Geometry check sheet. Reference: the model listing, model coordinates, mm. A direction names the side the tool comes from. Coordinates: 2 decimals unless noted, no trailing zeros. Write each loop counter-clockwise with the first axis right and the second up, starting at its lowest first coordinate (ties: lowest second). Pieces come first, ordered by that corner, then holes. Notation, with made-up numbers: (64.5, -14.75) -> (84.5, -14.75) arc R23 cw to (84.5, 24.25) -> close; hole circle Ø8 at (-20.75, 84). An arc over 180 degrees is marked (long way). Put each result on its own line as item: value. Start each with the question number.
from build123d import *

# Parameters (mm, degrees)
SKETCH1_W               = 21.5
SKETCH1_H               = 5
BOSS_EXTRUDE1_DEPTH     = 10
CUT_EXTRUDE1_DEPTH      = 75.426137882
CUT_EXTRUDE1_DEPTH_BACK = 75.426137882
SKETCH2_R               = 1.836585915
SKETCH3_W               = 21.5
SKETCH3_H               = 5
CUT_EXTRUDE2_DEPTH      = 10


with BuildPart() as part:
    # Sketch1 → Boss-Extrude1 (new body)
    with BuildSketch(Plane(origin=(0, 0, 0), x_dir=(0, 0, -1), z_dir=(1, 0, 0))):
        Polygon((-39, 10.5), (-39, -10.5), (39, -10.5), (39, 10.5), (34, 10.5), (34, -0.5), (34, -5.5), (12.5, -5.5), (-12.5, -5.5), (-34, -5.5), (-34, -0.5), (-34, 10.5), align=None)
        with Locations((-23.25, -3)):
            Rectangle(SKETCH1_W, SKETCH1_H)
        with Locations((23.25, -3)):
            Rectangle(SKETCH1_W, SKETCH1_H)
    extrude(amount=BOSS_EXTRUDE1_DEPTH)

    # Sketch2 → Cut-Extrude1 (cut, two sides: drawn at the far end of the back side and taken through both)
    with BuildSketch(Plane.XY.offset(-34).offset(-CUT_EXTRUDE1_DEPTH_BACK)):
        with Locations((5, 5)):
            Circle(SKETCH2_R)
    extrude(amount=CUT_EXTRUDE1_DEPTH + CUT_EXTRUDE1_DEPTH_BACK, mode=Mode.SUBTRACT)

    # Sketch3 → Cut-Extrude2 (cut)
    with BuildSketch(Plane(origin=(10, 0, 0), x_dir=(0, 0, -1), z_dir=(1, 0, 0))):
        with Locations((-28.25, -8)):
            Rectangle(SKETCH3_W, SKETCH3_H)
    cut_extrude2 = extrude(amount=-CUT_EXTRUDE2_DEPTH, mode=Mode.SUBTRACT)

    # Mirror1: Cut-Extrude2 across plane
    add(cut_extrude2.mirror(Plane.XY), mode=Mode.SUBTRACT)


solid = part.part
Item 1: Scan lines: line 1 along Z through (x, y) = (2.25, 8); line 2 along X through (y, z) = (5, -35.75); line 3 along Y through (x, z) = (5, 35.7). Record each from-to range of solid material in increasing order. Write a range as [from, to].
Item 2: Section check B-B, the plane x = 8.5. Enter the section's corners in (y, z).
Item 3: Section check D-D, the plane x = 5. Enter the section's corners in (y, z).
Item 4: Mould release check, pull along X, two halves, no side actions. Record for faces 1 (the flat face through (5, -5.5, -28)), 2 (the cylindrical face through (6.7, 4.3, 36.5)), 3 (the cylindrical face through (6.7, 4.3, -36.5)), 4 (the flat face through (10, -7, 1)): released by +X, released by -X, zero draft, split by the parting line, or undercut.
Item 5: Go/stop test with flat-tipped pins: P1, Ø5, axis at x = 3, z = -30.5, coming from the -Y side; P2, Ø5, axis at x = 4.5, y = 4.5, coming from the -Z side; P3, Ø1, axis at x = 7, z = 29, coming from the +Y side; P4, Ø2.5, axis at x = 4, y = -8.5, coming from the +Z side. Record where each tip stops, or that it passes through.
Item 6: Section check A-A, the plane y = -1.25. Enter the section's corners in (x, z).
Item 7: Section check C-C, the plane y = 5. Enter the section's corners in (x, z), and give its area (3 significant figures).
Item 8: Access from +Z, -Z, +X, -X, +Y, -Y to the whole of each face (thin tool, end or side, straight path). Record for faces 5 (the flat face through (5, -8, 17.5)), 6 (the flat face through (5, -10.5, 0)), 7 (the flat face through (3, 5, -34)).
From the geometry:
1. line 1: [-39, -34], [34, 39]
1. line 2: [0, 3.16], [6.84, 10]
1. line 3: [-5.5, 3.16], [6.84, 10.5]
2. outline: (-10.5, -17.5) -> (-5.5, -17.5) -> (-5.5, -39) -> (10.5, -39) -> (10.5, -34) -> (-0.5, -34) -> (-0.5, -12.5) -> (-5.5, -12.5) -> (-5.5, 12.5) -> (-0.5, 12.5) -> (-0.5, 34) -> (10.5, 34) -> (10.5, 39) -> (-5.5, 39) -> (-5.5, 17.5) -> (-10.5, 17.5) -> close
3. outline: (-10.5, -17.5) -> (-5.5, -17.5) -> (-5.5, -39) -> (3.16, -39) -> (3.16, -34) -> (-0.5, -34) -> (-0.5, -12.5) -> (-5.5, -12.5) -> (-5.5, 12.5) -> (-0.5, 12.5) -> (-0.5, 34) -> (3.16, 34) -> (3.16, 39) -> (-5.5, 39) -> (-5.5, 17.5) -> (-10.5, 17.5) -> close; (6.84, -39) -> (10.5, -39) -> (10.5, -34) -> (6.84, -34) -> close; (6.84, 34) -> (10.5, 34) -> (10.5, 39) -> (6.84, 39) -> close
4. face 1: zero draft
4. face 2: undercut
4. face 3: undercut
4. face 4: released by +X
5. P1: y = -5.5
5. P2: z = -39
5. P3: y = -0.5
5. P4: z = 17.5
6. outline: (0, -39) -> (10, -39) -> (10, -12.5) -> (0, -12.5) -> close; (0, 12.5) -> (10, 12.5) -> (10, 39) -> (0, 39) -> close
7. outline: (0, -39) -> (3.16, -39) -> (3.16, -34) -> (0, -34) -> close; (0, 34) -> (3.16, 34) -> (3.16, 39) -> (0, 39) -> close; (6.84, -39) -> (10, -39) -> (10, -34) -> (6.84, -34) -> close; (6.84, 34) -> (10, 34) -> (10, 39) -> (6.84, 39) -> close
7. area: 63.3 mm²
8. face 5: +Z, +X, -X, -Y
8. face 6: +Z, -Z, +X, -X, -Y
8. face 7: +X, -X, +Y
